Read the model definition and answer for the solid it produces. Units are mm, in the model's axes. Face numbers are marked on the shaded views. Coordinates: 2 decimals unless noted, no trailing zeros. Loops run counter-clockwise (first coordinate to the right, second up) from the corner with the lowest first, then second, coordinate; pieces in that order, holes last. Notation, with made-up numbers: (-23.5, 6.5) -> (3.5, 6.5) arc R13 ccw to (3.5, 29.5) -> close; hole circle Ø6 at (19, 43). An arc over 180 degrees is marked (long way). Answer as a JSON object with one key per item and string values. Group by question number.
Q1. The part is cut by section C-C on z = -44. Write down the section's boundary in (x, y).
Q2. The part is cut by section B-B on x = 2.5. Write down the section's boundary in (y, z), and give its area (3 significant figures).
Q3. The part is cut by section A-A on z = -17.5. Write down the section's boundary in (x, y), and give its area (3 significant figures).
Q4. Each of these flat-tipped pins is pushed along its axis until it touches: P1, Ø2, axis at x = -23, y = 3, coming from the -Z side; P2, Ø1, axis at x = -26, y = 5, coming from the +Z side; P3, Ø3, axis at y = 4.5, z = -29.5, coming from the -X side; P4, Ø3, axis at x = -5.5, y = 3.5, coming from the +Z side. Where does it stop, or does it pass through?
Q5. Determine the mould class of the marked faces 1 and 2 for opening direction Z: released by +Z, released by -Z, zero draft, split by the parting line, or undercut.
Q6. Straight lines are drawn through the part: line 1 along X through (y, z) = (1.25, -23); line 2 along Y through (x, z) = (28, -31); line 3 along X through (y, z) = (2, -24). For each, find the intervals that lie inside material, in ascending order. Write a range as [from, to].
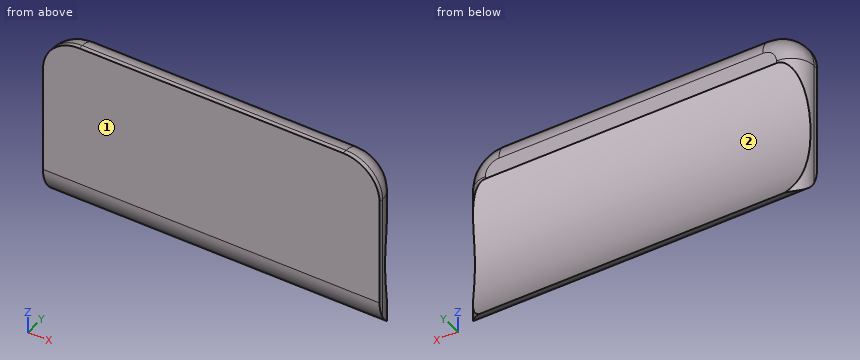
Autodesk Inventor part; units mm, degrees
ref_plane "YZ Plane" through (0, 0, 0) normal (1, 0, 0) x (0, 1, 0)
ref_plane "XZ Plane" through (0, 0, 0) normal (0, 1, 0) x (-1, 0, 0)
ref_plane "XY Plane" through (0, 0, 0) normal (0, 0, 1) x (1, 0, 0)
sketch "Sketch1" plane through (0, 0, 0) normal (0, 1, 0) x (-1, 0, 0)
  line L0 (25.9, 0) -> (-25.9, 0)
  line L1 (0, -25.9) -> (0, 25.9)
  circle A0 centre (0, 0) radius 18.5 construction
  circle A1 centre (0, 0) radius 13 construction
  dimension "d0" = 37
  dimension "d1" = 26
sketch "Sketch2" plane through (0, 0, 0) normal (0, 1, 0) x (-1, 0, 0)
  line L0 (0, -28.9) -> (0, 26.4)
  line L1 (-37, -8) -> (-37, -21)
  line L2 (-37, -21) -> (37, -21)
  line L3 (37, -21) -> (37, -8)
  line L4 (37, -8) -> (-37, -8)
  line L5 (-51.8, 0) -> (51.8, 0)
  point P0 (0, 0)
  dimension "d3" = 74
  dimension "d99" = 8
  dimension "d101" = 21
extrude "Extrusion1" add sketch "Sketch2" along normal blind 6
sketch "Sketch6" plane through (0, 0, 0) normal (0, 1, 0) x (-1, 0, 0)
  line L0 (37, -21) -> (-37, -21)
  line L1 (37, -8) -> (37, -21)
  line L2 (-37, -21) -> (37, -21)
  line L3 (37, -21) -> (37, -8)
  line L4 (-37, -8) -> (-37, -21)
  line L5 (58.8, 0) -> (-58.8, 0)
  line L6 (0, -28.9) -> (0, 26.4)
  arc A0 (-16, 0) -> (16, 0) centre (0, 0) ccw
  line L7 (16, 0) -> (16, 0)
  line L8 (37, 0) -> (-37, 0)
  line L9 (16, 0) -> (37, 0)
  line L10 (-16, 0) -> (-16, 0)
  line L11 (-16, 0) -> (-37, 0)
  point P0 (-17.3617, -21)
  dimension "d18" = 32
extrude "Extrusion5" [suppressed]
sketch "Sketch4" plane through (0, 0, 0) normal (0, 0, 1) x (1, 0, 0)
  line L0 (-18.5, 0) -> (18.5, 0)
  line L1 (18.5, 0) -> (18.5, -2)
  line L2 (18.5, -2) -> (-18.5, -2)
  line L3 (-18.5, -2) -> (-18.5, 0)
  line L4 (-25.9, 0) -> (25.9, 0)
  line L5 (0, -2.4) -> (0, 0.4)
  point P0 (0, 0)
  dimension "d10" = 37
  dimension "d11" = 2
extrude "Extrusion6" [suppressed]
sketch "Sketch5" plane through (0, 0, 0) normal (0, 1, 0) x (-1, 0, 0)
  circle A0 centre (0, 0) radius 18.5 construction
  circle A1 centre (0, 0) radius 18.5 construction
  line L0 (25.9, 0) -> (-25.9, 0)
  line L1 (0, -28.9) -> (0, 26.4)
  line L2 (-18.5, -21) -> (18.5, -21)
  line L3 (18.5, -21) -> (18.5, -18.5)
  line L4 (18.5, -18.5) -> (-18.5, -18.5)
  line L5 (-18.5, -18.5) -> (-18.5, -21)
  dimension "d25" = 37
  dimension "d26" = 21
extrude "Extrusion7" [suppressed]
sketch "Sketch7" plane through (0, 0, 0) normal (0, 0, 1) x (1, 0, 0)
  line L0 (-18.5, 0) -> (18.5, 0)
  line L1 (18.5, 0) -> (18.5, -2)
  line L2 (18.5, -2) -> (-18.5, -2)
  line L3 (-18.5, -2) -> (-18.5, 0)
  line L4 (37, 0) -> (-37, 0)
  line L5 (-58.8, 0) -> (58.8, 0)
  line L6 (0, -2.4) -> (0, 0.4)
  point P0 (-16, 0)
  point P1 (16, 0)
  dimension "d53" = 2
  dimension "d54" = 18.5
extrude "Extrusion8" [suppressed]
sketch "Sketch8" plane through (0, 0, 0) normal (0, 1, 0) x (-1, 0, 0)
  circle A0 centre (0, 0) radius 12.75
  dimension "d34" = 25.5
extrude "Extrusion9" [suppressed]
pattern_linear "Rectangular Pattern1" [suppressed]
sketch "Sketch9" plane through (0, 6, 0) normal (0, 1, 0) x (1, 0, 0)
  circle A0 centre (0, 0) radius 13
  circle A1 centre (0, 0) radius 15
  dimension "d40" = 26
  dimension "d41" = 30
extrude "Extrusion10" [suppressed]
sketch "Sketch10" plane through (0, 5, 0) normal (0, 1, 0) x (1, 0, 0)
  arc A0 (16, 0) -> (-16, 0) centre (0, 0) ccw
  line L0 (1.5, -18) -> (-1.5, -18)
  line L1 (-29.4, 0) -> (29.4, 0)
  line L2 (0, 36.3) -> (0, -70.8)
  line L3 (1.5, -12) -> (-1.5, -12)
  line L4 (1.5, -12) -> (1.5, -18)
  line L5 (-1.5, -18) -> (-1.5, -12)
  dimension "d48" = 3
  dimension "d49" = 12
  dimension "d50" = 6
extrude "Extrusion11" [suppressed]
fillet "Fillet1" [suppressed]
sketch "Sketch11" plane through (0, 0, 0) normal (0, 1, 0) x (-1, 0, 0)
  line L0 (-37, -21) -> (37, -21)
  line L1 (37, -21) -> (37, -47)
  line L2 (37, -47) -> (-37, -47)
  line L3 (-37, -47) -> (-37, -21)
  line L4 (58.8, 0) -> (-58.8, 0)
  line L5 (0, -60.1) -> (0, 31.6)
  point P0 (0, 0)
  dimension "d57" = 26
  dimension "d58" = 21
  dimension "d59" = 74
extrude "Extrusion12" add sketch "Sketch11" along normal blind 6
sketch "Sketch12" plane through (0, 0, 0) normal (1, 0, 0) x (0, 1, 0)
  line L0 (6, -8) -> (6, -47)
  arc A0 (6, -16.5081) -> (5.7334, -47) centre (34, -32) ccw
  line L1 (-6.8, 0) -> (40.8, 0)
  line L2 (0, -66) -> (0, 67)
  line L3 (6, -16.5081) -> (6, -47)
  line L4 (6, -47) -> (5.7334, -47)
  line L5 (0, -47) -> (6, -47)
  point P0 (0, 0)
  point P1 (6, 48)
  dimension "d62" = 32
  dimension "d63" = 32
  dimension "d64" = 34
extrude "Extrusion13" cut sketch "Sketch12" along normal through all both and the other way through all
fillet "Fillet3" radius 8 1 edges at (0, 0, -47)
sketch "Sketch13" plane through (0, 0, 0) normal (0, 1, 0) x (-1, 0, 0)
  line L0 (61.5, 0) -> (-75, 0)
  line L1 (0, -57.9802) -> (0, 72.5866)
  line L2 (37, -8) -> (37, -39.3278)
  arc A0 (13.0815, 23.9185) -> (13.0815, 13.0815) centre (18.5, 18.5) ccw
  line L3 (-37, -8) -> (-37, -16.5081)
  arc A1 (-13.0815, 13.0815) -> (-13.0815, 23.9185) centre (-18.5, 18.5) ccw
  line L4 (18.5, 37) -> (18.5, 0)
  line L5 (-18.5, 0) -> (-18.5, 37)
  line L6 (18.5, 37) -> (18.5, -8)
  line L7 (-37, 0) -> (37, 0)
  line L8 (-18.5, -8) -> (-18.5, 37)
  arc A2 (-9.2871, 53) -> (-13.0815, 23.9185) centre (0, 37) ccw
  arc A3 (13.0815, 23.9185) -> (9.2871, 53) centre (0, 37) ccw
  arc A4 (-13.0815, 13.0815) -> (-18.5, 0) centre (0, 0) ccw
  arc A5 (18.5, 0) -> (13.0815, 13.0815) centre (0, 0) ccw
  point P0 (37, -39.3278)
  point P1 (-55.5, 48)
  point P2 (-37, -16.5081)
  dimension "d68" = 37
  dimension "d71" = 18.5
  dimension "d72" = 18.5
  dimension "d73" = 7.663
  dimension "d74" = 7.663
  dimension "d75" = 18.5
  dimension "d76" = 18.5
  dimension "d77" = 18.5
  dimension "d78" = 18.5
extrude "Extrusion14" [suppressed]
sketch "Sketch14" plane through (0, 0, 0) normal (0, 1, 0) x (-1, 0, 0)
  circle A0 centre (18.5, 18.5) radius 10
  line L0 (39.9, 0) -> (-39.9, 0)
  line L1 (0, -27.9) -> (0, 37.9)
  circle A1 centre (-18.5, 18.5) radius 10
  point P0 (0, 0)
  dimension "d84" = 18.5
  dimension "d85" = 18.5
  dimension "d86" = 20
  dimension "d89" = 37
extrude "Extrusion15" [suppressed]
fillet "Fillet4" [suppressed]
fillet "Fillet5" radius 8 2 edges at (-37, 3, -8) (37, 3, -8)
fillet "Fillet6" radius 5 5 edges at (34.6569, 6, -10.3431) (37, 6, -16.254) (-34.6569, 6, -10.3431) (-37, 6, -16.254) (0, 6, -8)
equation "\"d85\" = d84"
properties part number "NespressoSpeedfiller-6X-long-scraper"
Final values:
{
 "1": {"outline": "(-36.97, 1.51) -> (36.97, 1.51) arc R5 ccw to (35.73, 4.34) -> (-35.73, 4.34) arc R5 ccw to start"},
 "2": {"outline": "(0, -39.33) arc R8 ccw to (5.73, -47) arc R32 cw to (6, -16.51) -> (6, -13) arc R5 ccw to (1, -8) -> (0, -8) -> close", "area": "133 mm2"},
 "3": {"outline": "(-37, 0) -> (37, 0) -> (37, 1) arc R5 ccw to (34.23, 5.47) -> (-34.23, 5.47) arc R5 ccw to (-37, 1) -> close", "area": "398 mm2"},
 "4": {"P1": "stops at z = -46.26", "P2": "stops at z = -9.43", "P3": "passes through", "P4": "stops at z = -8.1"},
 "5": {"face 1": "zero draft", "face 2": "undercut"},
 "6": {"line 1": "x = [-36.99, 36.99]", "line 2": "y = [0, 2.02]", "line 3": "x = [-36.9, 36.9]"}
}
